CAD build for the part. Positions are in the model's coordinates, mm. A direction names the side the tool comes from. Coordinates: 2 decimals unless noted, no trailing zeros. Loops run counter-clockwise (first coordinate to the right, second up) from the corner with the lowest first, then second, coordinate; pieces in that order, holes last. Notation, with made-up numbers: (51.5, 2.5) -> (67.5, 2.5) arc R26 cw to (67.5, 37.5) -> close; hole circle Ø6 at (-10, -4). An arc over 180 degrees is marked (long way). Return JSON: item names as keys, results as strings. Group by question number.
(1) Tool access for faces 1 (the face through (0, 0, 155.9)), 2 (the face through (-18, 0, 120.4)): list every direction of +Z, -Z, +X, -X, +Y, -Y with a clear straight run to the whole face (end or side of a thin tool).
(2) Saw through at B-B on z = 135.5. Write the cut outline in (x, y).
(3) Saw through at A-A on z = 66. Write the cut outline in (x, y), then the cut area to 3 significant figures.
(4) Mould opens along X. For faces 3 (the face through (20.03, 6.31, 98.31)), 4 (the face through (15.9, -1.2, 123.4)), 5 (the face through (2, 0, -1.35)) say: pulls with the +X half, pulls with the -X half, needs draft (parallel to the pull), parting line crosses it, or undercut.
(5) Flat gauge pins, fed straight in: pin 1 Ø3 at (x, y) = (-17.5, 0) entering from -Z; pin 2 Ø1 at (x, y) = (2, 15) entering from -Z; pin 3 Ø1.3 at (x, y) = (-10.21, 7.55) entering from +Z. Where does each tip first touch, or does it go through?
(6) Probe L1, parallel to Z at x = 12, y = -8.5; L2, parallel to X at y = -0.5, z = 77; L3, parallel to Z at x = -5.5, y = -4. List the from-to ranges inside material, lowest first.
```python
from build123d import *

# Parameters (mm, degrees)
ESQUISSE1_R             = 20
BOSS_EXTRU_1_DEPTH      = 71
ESQUISSE2_R             = 4
BOSS_EXTRU_2_DEPTH      = 1.35
ESQUISSE3_R             = 1.5
BOSS_EXTRU_3_DEPTH      = 15.7
ESQUISSE11_R            = 20.05
BOSS_EXTRU_8_DEPTH      = 3
ESQUISSE12_R            = 1
ESQUISSE12_R_2          = 0.8
ENL_V_MAT_EXTRU_4_DEPTH = 1
ESQUISSE4_R             = 21
BOSS_EXTRU_9_DEPTH      = 55.4
ESQUISSE13_R            = 14
BOSS_EXTRU_10_DEPTH     = 3
ESQUISSE14_R            = 6
BOSS_EXTRU_11_DEPTH     = 26.5
ESQUISSE15_R            = 2
ENL_V_MAT_EXTRU_5_DEPTH = 6


with BuildPart() as part:
    # Esquisse1 → Boss.-Extru.1 (new body)
    with BuildSketch(Plane.XY):
        Circle(ESQUISSE1_R)
    extrude(amount=BOSS_EXTRU_1_DEPTH)

    # Esquisse2 → Boss.-Extru.2 (add)
    with BuildSketch(Plane(origin=(0, 0, 0), x_dir=(-1, 0, 0), z_dir=(0, 0, -1))):
        with Locations(Location((0, 0, 0), (0, 0, 180))):
            Circle(ESQUISSE2_R)
    extrude(amount=BOSS_EXTRU_2_DEPTH)

    # Esquisse3 → Boss.-Extru.3 (add)
    with BuildSketch(Plane(origin=(0, 0, 0), x_dir=(-1, 0, 0), z_dir=(0, 0, -1))):
        Circle(ESQUISSE3_R)
    extrude(amount=BOSS_EXTRU_3_DEPTH)

    # Esquisse11 → Boss.-Extru.8 (add)
    with BuildSketch(Plane(origin=(0, 0, 0), x_dir=(-1, 0, 0), z_dir=(0, 0, -1))):
        Circle(ESQUISSE11_R)
    extrude(amount=-BOSS_EXTRU_8_DEPTH)

    # Esquisse12 → Enlèv. mat.-Extru.4 (cut)
    with BuildSketch(Plane(origin=(0, 0, 0), x_dir=(-1, 0, 0), z_dir=(0, 0, -1))):
        with Locations((1.720688849, -15.102292206)):
            Circle(ESQUISSE12_R)
        with Locations((-1.720688849, 15.102292206)):
            Circle(ESQUISSE12_R)
        with Locations((-12.218624281, -9.041306359)):
            Circle(ESQUISSE12_R)
        with Locations((10.20898213, 7.554249392)):
            Circle(ESQUISSE12_R_2)
        with Locations((-10.20898213, -7.554249392)):
            Circle(ESQUISSE12_R_2)
        with Locations((-9.041306359, 12.218624281)):
            Circle(ESQUISSE12_R)
        with Locations((12.218624281, 9.041306359)):
            Circle(ESQUISSE12_R)
        with Locations((9.041306359, -12.218624281)):
            Circle(ESQUISSE12_R)
        Polygon((13.553659243, -1.043501598), (19.3492142, -2.596415868), (18.055118975, -7.426045), (12.259564017, -5.873130729), align=None)
        Polygon((-13.584662099, -0.497523966), (-19.51875728, 0.389332501), (-18.779710224, 5.334411818), (-12.845615044, 4.447555351), align=None)
    extrude(amount=-ENL_V_MAT_EXTRU_4_DEPTH, mode=Mode.SUBTRACT)

    # Esquisse4 → Boss.-Extru.9 (add)
    with BuildSketch(Plane.XY.offset(71)):
        Circle(ESQUISSE4_R)
    extrude(amount=BOSS_EXTRU_9_DEPTH)

    # Esquisse13 → Boss.-Extru.10 (add)
    with BuildSketch(Plane.XY.offset(126.4)):
        Circle(ESQUISSE13_R)
    extrude(amount=BOSS_EXTRU_10_DEPTH)

    # Esquisse14 → Boss.-Extru.11 (add)
    with BuildSketch(Plane.XY.offset(129.4)):
        Circle(ESQUISSE14_R)
    extrude(amount=BOSS_EXTRU_11_DEPTH)

    # Esquisse15 → Enlèv. mat.-Extru.5 (cut)
    with BuildSketch(Plane.XY.offset(126.4)):
        with Locations((0, -17.5)):
            Circle(ESQUISSE15_R)
        with Locations((-17.5, 0)):
            Circle(ESQUISSE15_R)
        with Locations((0, 17.5)):
            Circle(ESQUISSE15_R)
        with Locations((17.5, 0)):
            Circle(ESQUISSE15_R)
    extrude(amount=-ENL_V_MAT_EXTRU_5_DEPTH, mode=Mode.SUBTRACT)


solid = part.part
```
Geometry results:
{
 "1": {"face 1": "+Z, +X, -X, +Y, -Y", "face 2": "+Z"},
 "2": {"outline": "circle Ø12 at (0, 0)"},
 "3": {"outline": "circle Ø40 at (0, 0)", "area": "1,260 mm²"},
 "4": {"face 3": "parting line crosses it", "face 4": "undercut", "face 5": "needs draft"},
 "5": {"pin 1": "z = 0", "pin 2": "z = 1", "pin 3": "z = 129.4"},
 "6": {"L1": "1 to 126.4", "L2": "-20.99 to 20.99", "L3": "0 to 129.4"}
}
